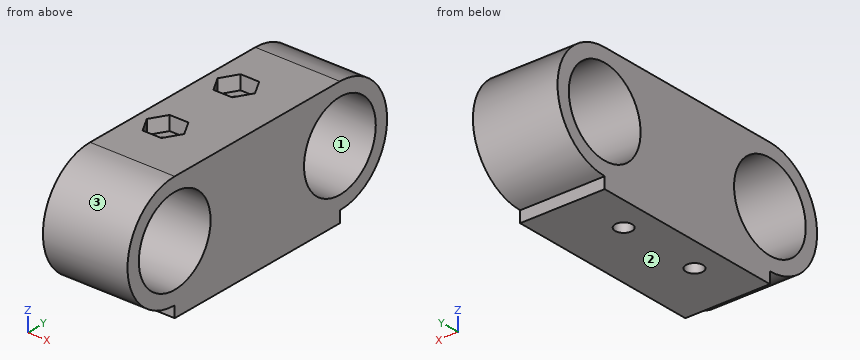
```python
from build123d import *

# Parameters (mm, degrees)
SKETCH039_R          = 7.6
PAD012_DEPTH         = 15
SKETCH040_R          = 1.5
POCKET024_DEPTH      = 10.001
POCKET024_DEPTH_BACK = 12.001
POCKET025_DEPTH      = 2.5


with BuildPart() as part:
    # Sketch039 → Pad012 (new body)
    with BuildSketch(Plane.YZ):
        with BuildLine():
            Line((-17.5, 10), (17.5, 10))
            ThreePointArc((17.5, -10), (27.5, 0), (17.5, 10))
            Line((17.5, -12), (17.5, -10))
            Line((-17.5, -12), (17.5, -12))
            Line((-17.5, -10), (-17.5, -12))
            ThreePointArc((-17.5, 10), (-27.5, 0), (-17.5, -10))
        make_face()
        with Locations((17.5, 0)):
            Circle(SKETCH039_R, mode=Mode.SUBTRACT)
        with Locations((-17.5, 0)):
            Circle(SKETCH039_R, mode=Mode.SUBTRACT)
    extrude(amount=PAD012_DEPTH)

    # Sketch040 → Pocket024 (cut, two sides)
    with BuildSketch(Plane.XY) as pocket024_sk:
        with Locations((5, 7.5)):
            Circle(SKETCH040_R)
        with Locations((5, -7.5)):
            Circle(SKETCH040_R)
    extrude(amount=POCKET024_DEPTH, mode=Mode.SUBTRACT)
    extrude(pocket024_sk.sketch, amount=-POCKET024_DEPTH_BACK, mode=Mode.SUBTRACT)

    # Sketch041 → Pocket025 (cut)
    with BuildSketch(Plane.XY.offset(10)):
        Polygon((6.6575, 10.3708742135), (3.3425, 10.3708742135), (1.685, 7.5), (3.3425, 4.6291257865), (6.6575, 4.6291257865), (8.315, 7.5), align=None)
        Polygon((6.6575, -4.6291257865), (3.3425, -4.6291257865), (1.685, -7.5), (3.3425, -10.3708742135), (6.6575, -10.3708742135), (8.315, -7.5), align=None)
    extrude(amount=-POCKET025_DEPTH, mode=Mode.SUBTRACT)


with BuildPart() as part_1:
    # Body007 placement: moved
    add(part.part.moved(Location((30, 0, -50))))


solid = part_1.part
```
The model under review builds one solid part; all positions refer to its coordinate system, in mm. Face numbers are marked on the shaded views. Round coordinates to 2 decimals unless told otherwise and drop trailing zeros. Order: outer loops, then holes, each group sorted by start corner. A loop starts at its lowest first (then second) coordinate and runs counter-clockwise, first axis right, second up. Notation, with made-up numbers: M 12,30 L 71,30 A19 ccw 71,39 Z; hole C 68,24 d3. An arc over 180 degrees is marked long. Use a Markdown table: item, result.
1) Consider section D-D (z = -41.5). Write out the cut boundary in (x, y) (1 decimal), then the cut area to 3 significant figures.
Report:
| item | result |
|---|---|
| outline | M 30,-22.8 L 45,-22.8 L 45,22.8 L 30,22.8 Z; hole M 31.7,-7.5 L 33.3,-10.4 L 36.7,-10.4 L 38.3,-7.5 L 36.7,-4.6 L 33.3,-4.6 Z; hole M 31.7,7.5 L 33.3,4.6 L 36.7,4.6 L 38.3,7.5 L 36.7,10.4 L 33.3,10.4 Z |
| area | 626 mm^2 |
2) Insertion check: pin 1 (0.8 mm diameter, centred on x = 34.5, z = -41, fed in from +Y); pin 2 (3 mm diameter, centred on y = 21, z = -56.5, fed in from +X); pin 3 (1.2 mm diameter, centred on x = 35, z = -42, fed in from +Y); pin 4 (1 mm diameter, centred on x = 34, z = -61, fed in from +Y). Each pin has a flat end and moves straight along its axis. Give the tip position at first contact, or say it passes through.
Report:
| item | result |
|---|---|
| pin 1 | y = 22.6 |
| pin 2 | x = 45 |
| pin 3 | y = 24.23 |
| pin 4 | y = 17.5 |
3) Consider section C-C (y = -13). Write out the cut boundary in (x, z).
Report:
| item | result |
|---|---|
| outline | M 30,-62 L 45,-62 L 45,-56.12 L 30,-56.12 Z; M 30,-43.88 L 45,-43.88 L 45,-40 L 30,-40 Z |
4) Wall thickness on line 1 along Y through (x, z) = (31.25, -53.5); line 2 along X through (y, z) = (7.5, -47.25); line 3 along Y through (x, z) = (35, -54.75): over which ranges is each line inside the solid? List them lowest first. Write a range as [from, to].
Report:
| item | result |
|---|---|
| line 1 | [-26.87, -24.25], [-10.75, 10.75], [24.25, 26.87] |
| line 2 | [30, 33.5], [36.5, 45] |
| line 3 | [-26.3, -23.43], [-11.57, -9], [-6, 6], [9, 11.57], [23.43, 26.3] |
5) Draft analysis for pull direction Z (two halves, no side actions). For the marked faces 1, 2 and 3, state which applies: released by +Z, released by -Z, zero draft, split by the parting line, or undercut.
Report:
| item | result |
|---|---|
| face 1 | undercut |
| face 2 | released by -Z |
| face 3 | split by the parting line |
6) Consider section A-A (x = 35). Write out the cut boundary in (y, z).
Report:
| item | result |
|---|---|
| outline | M -17.5,-62 L -9,-62 L -9,-42.5 L -10.37,-42.5 L -10.37,-40 L -17.5,-40 A10 ccw -17.5,-60 Z; M -6,-62 L 6,-62 L 6,-42.5 L 4.63,-42.5 L 4.63,-40 L -4.63,-40 L -4.63,-42.5 L -6,-42.5 Z; M 9,-62 L 17.5,-62 L 17.5,-60 A10 ccw 17.5,-40 L 10.37,-40 L 10.37,-42.5 L 9,-42.5 Z; hole C -17.5,-50 d15.2; hole C 17.5,-50 d15.2 |
7) Consider section B-B (z = -44.75). Write out the cut boundary in (x, y).
Report:
| item | result |
|---|---|
| outline | M 30,-26.01 L 45,-26.01 L 45,-23 L 30,-23 Z; M 30,-12 L 45,-12 L 45,12 L 30,12 Z; M 30,23 L 45,23 L 45,26.01 L 30,26.01 Z; hole C 35,-7.5 d3; hole C 35,7.5 d3 |
